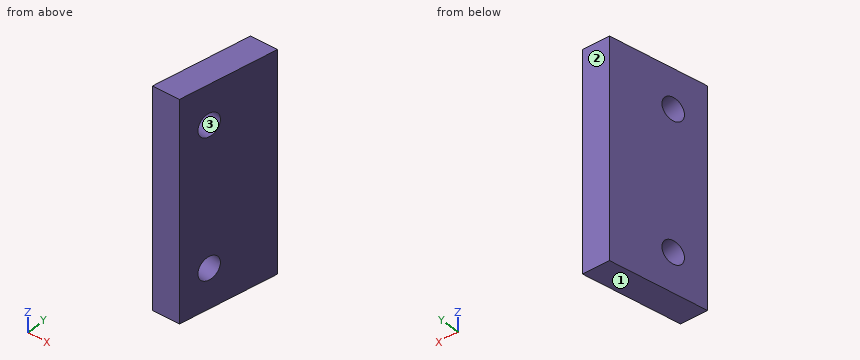
```python
from build123d import *

# Parameters (mm, degrees)
BOSS_EXTRUDE2_DEPTH = 20
SKETCH4_R           = 1.05
CUT_EXTRUDE1_DEPTH  = 5.024852982


with BuildPart() as part:
    # Sketch2 → Boss-Extrude2 (new body)
    with BuildSketch(Plane.XY):
        Polygon((0, 0), (2.5, 0), (4.086942826, 9), (1.586942826, 9), align=None)
    extrude(amount=BOSS_EXTRUDE2_DEPTH)

    # Sketch4 → Cut-Extrude1 (cut, through all)
    with BuildSketch(Plane(origin=(0, 0, 0), x_dir=(0, 0, 1), z_dir=(-0.984807753, 0.173648178, 0))):
        with Locations((3.625, 3.2)):
            Circle(SKETCH4_R)
        with Locations((16.375, 3.2)):
            Circle(SKETCH4_R)
    extrude(amount=-CUT_EXTRUDE1_DEPTH, mode=Mode.SUBTRACT)


solid = part.part
```
Could you check a few things on this model? Use its own coordinates, in mm. Face numbers are marked on the shaded views. Give positions to 0.01 mm unless a question says otherwise; leave off trailing zeros. Loops run counter-clockwise (first coordinate to the right, second up) from the corner with the lowest first, then second, coordinate; pieces in that order, holes last. Notation, with made-up numbers: (64.25, 83) - (83.25, 83) arc R22 cw to (83.25, 98) - close; hole circle Ø8 at (21.25, 18). An arc over 180 degrees is marked (long way). Answer in a Markdown table with one row per item. Add a question column.
Q1. For pin 1 (4 mm diameter, centred on y = 5.5, z = 16, fed in from -X); pin 2 (3 mm diameter, centred on y = 6.5, z = 6.5, fed in from -X), each with a flat end and sliding along its axis, tell me the tip position at first contact or that it passes through.
Q2. If we section it at D-D (y = 6): List the corners of the cut face in (x, z) for me.
Q3. If we section it at C-C (x = 1.35): State how many separate pieces and enclosed holes the cut face has, plus the area to 3 significant figures.
Q4. Please list where these lines run through material, in increasing order: L1, parallel to Z at x = 2, y = 3.25; L2, parallel to Z at x = 1.25, y = 3.5; L3, parallel to X at y = 8.5, z = 18.75. Write a range as from..to.
Q5. If we section it at A-A (z = 3.5): List the corners of the cut face in (x, y) for me.
Q6. If we section it at B-B (z = 6): List the corners of the cut face in (x, y) for me.
Q7. We'd pull the mould along Z, two halves only. Please class the marked faces 1, 2 and 3: +Z half, -Z half, draft (parallel to the pull), parting line (faces both ways), or undercut.
The answers:
| question | item | result |
|---|---|---|
| 1 | pin 1 | stops at x = 0.63 |
| 1 | pin 2 | stops at x = 0.88 |
| 2 | outline | (1.06, 0) - (3.56, 0) - (3.56, 20) - (1.06, 20) - close |
| 3 | separate pieces | 1 |
| 3 | enclosed holes | 2 |
| 3 | area | 146 mm^2 |
| 4 | L1 | z = 0..2.63, 4.62..15.38, 17.37..20 |
| 4 | L2 | z = 0..2.68, 4.57..15.43, 17.32..20 |
| 4 | L3 | x = 1.5..4 |
| 5 | outline | (0, 0) - (2.5, 0) - (2.8, 1.7) - (0.37, 2.12) - close; (0.74, 4.18) - (3.16, 3.75) - (4.09, 9) - (1.59, 9) - close |
| 6 | outline | (0, 0) - (2.5, 0) - (4.09, 9) - (1.59, 9) - close |
| 7 | face 1 | -Z half |
| 7 | face 2 | draft |
| 7 | face 3 | undercut |
